Here's how the part is built. I have some questions about the finished solid (model axes, mm). A direction names the side the tool comes from. Round coordinates to 2 decimals unless told otherwise and drop trailing zeros. Loops run counter-clockwise (first coordinate to the right, second up) from the corner with the lowest first, then second, coordinate; pieces in that order, holes last. Notation, with made-up numbers: (35.25, 53) -> (77.25, 53) arc R22 ccw to (77.25, 68) -> close; hole circle Ø5 at (70, 4.5). An arc over 180 degrees is marked (long way). Use CSV: the item, a comma, the result in double quotes. Start each with the question number.
from build123d import *

# Parameters (mm, degrees)
F0_W     = 10.2
F0_H     = 10.2
F0_W_2   = 32
F0_H_2   = 26
F0_W_3   = 6
F0_H_3   = 6
F0_W_4   = 8
F0_H_4   = 7
F0_H_5   = 1
F1_DEPTH = 2
F2_DEPTH = 8.5
F3_DEPTH = 10.2
F4_DEPTH = 25
F6_DEPTH = 5.5


with BuildPart() as f1:
    # F0 (on Right) → F1 (new body)
    with BuildSketch(Plane.YZ):
        Polygon((0, 55), (0, 26), (32, 26), (32, 55), (30, 55), (30, 48), (22, 48), (22, 55), align=None)
        with Locations((21.9, 39.9)):
            Rectangle(F0_W, F0_H, mode=Mode.SUBTRACT)
        with Locations((16, 13)):
            Rectangle(F0_W_2, F0_H_2)
        with Locations((6.6, 12)):
            Rectangle(F0_W_3, F0_H_3, mode=Mode.SUBTRACT)
        with Locations((25.4, 12)):
            Rectangle(F0_W_3, F0_H_3, mode=Mode.SUBTRACT)
        Polygon((0, 60), (0, 55), (22, 55), (22, 56), (30, 56), (30, 55), (32, 55), (32, 60), align=None)
        with Locations((21.9, 39.9)):
            Rectangle(F0_W, F0_H)
        with Locations((26, 51.5)):
            Rectangle(F0_W_4, F0_H_4)
        with Locations((25.4, 12)):
            Rectangle(F0_W_3, F0_H_3)
        with Locations((6.6, 12)):
            Rectangle(F0_W_3, F0_H_3)
        with Locations((26, 55.5)):
            Rectangle(F0_W_4, F0_H_5)
    extrude(amount=F1_DEPTH)

    # F0 (on Right) → F2 (join)
    with BuildSketch(Plane.YZ):
        Polygon((0, 55), (0, 26), (32, 26), (32, 55), (30, 55), (30, 48), (22, 48), (22, 55), align=None)
        with Locations((21.9, 39.9)):
            Rectangle(F0_W, F0_H, mode=Mode.SUBTRACT)
        with Locations((26, 51.5)):
            Rectangle(F0_W_4, F0_H_4)
        with Locations((21.9, 39.9)):
            Rectangle(F0_W, F0_H)
    extrude(amount=-F2_DEPTH)

    # F0 (on Right) → F4 (join)
    with BuildSketch(Plane.YZ):
        with Locations((26, 51.5)):
            Rectangle(F0_W_4, F0_H_4)
        with Locations((26, 55.5)):
            Rectangle(F0_W_4, F0_H_5)
    extrude(amount=F4_DEPTH)


with BuildPart() as f3:
    # F0 (on Right) → F3 (new body)
    with BuildSketch(Plane.YZ):
        with Locations((21.9, 39.9)):
            Rectangle(F0_W, F0_H)
    extrude(amount=F3_DEPTH)

    # F5: union F1
    add(f1.part)

    # F0 (on Right) → F6 (join)
    with BuildSketch(Plane.YZ):
        with Locations((6.6, 12)):
            Rectangle(F0_W_3, F0_H_3)
        with Locations((25.4, 12)):
            Rectangle(F0_W_3, F0_H_3)
    extrude(amount=-F6_DEPTH)


solid = f3.part
Q1. Will these pins go through, and if not, where does the flat tip stop? pin 1 Ø1.6 at (x, y) = (-3.5, 26.5) entering from +Z; pin 2 Ø2.5 at (y, z) = (22, 58.5) entering from -X; pin 3 Ø3 at (y, z) = (13.5, 53) entering from +X; pin 4 Ø1.5 at (x, z) = (11, 40.5) entering from +Y.
Q2. For faces 4 (the flat face through (-3, 25, 9)), 5 (the flat face through (6, 16.8, 40)), 6 (the flat face through (-3, 3.6, 12)), 7 (the flat face through (-4, 16, 26)), 8 (the flat face through (10.2, 22, 40)), which set-ups out of +Z, -Z, +X, -X, +Y, -Y let a thin tool reach every point of the face, with its end or its side?
Q3. I want a section at C-C, the plane y = 18.5. List the corners of the cut face in (x, z) for me, then the cut area to 3 significant figures.
Q4. I want a section at B-B, the plane z = 50. List the corners of the cut face in (x, y) for me, then the cut area to 3 significant figures.
Q5. I need wall thicknesses on line 1 along Z through (x, y) = (-3, 28); line 2 along X through (y, z) = (6.5, 11.5); line 3 along X through (y, z) = (15, 25). Which ranges of each line are inside material? Lowest first, please.
Q6. I want a section at D-D, the plane z = 13. List the corners of the cut face in (x, y) for me.
Q7. I want a section at A-A, the plane x = 3. List the corners of the cut face in (y, z) for me, then the cut area to 3 significant figures.
Q8. If we mould it in two halves opening along Z, with no side actions, what happens to faces 1 (the flat face through (-3, 7, 15)), 2 (the flat face through (-5.5, 7, 12)), 3 (the flat face through (6, 22, 34.8))? For each: pulls with the +Z half, pulls with the -Z half, needs draft (parallel to the pull), parting line crosses it, or undercut.
Values found:
1,pin 1,"z = 55"
1,pin 2,"x = 0"
1,pin 3,"x = 2"
1,pin 4,"through"
2,face 4,"-Z, -X, +Y, -Y"
2,face 5,"+Z, -Z, +X, -Y"
2,face 6,"-Z, -X, -Y"
2,face 7,"-X, +Y, -Y"
2,face 8,"-Z, +X, +Y, -Y"
3,outline,"(-8.5, 26) -> (0, 26) -> (0, 0) -> (2, 0) -> (2, 34.8) -> (10.2, 34.8) -> (10.2, 45) -> (2, 45) -> (2, 60) -> (0, 60) -> (0, 55) -> (-8.5, 55) -> close"
3,area,"450 mm2"
4,outline,"(-8.5, 0) -> (2, 0) -> (2, 22) -> (25, 22) -> (25, 30) -> (2, 30) -> (2, 32) -> (-8.5, 32) -> close"
4,area,"520 mm2"
5,line 1,"9 to 15, 26 to 55"
5,line 2,"-5.5 to 2"
5,line 3,"0 to 2"
6,outline,"(-5.5, 3.6) -> (0, 3.6) -> (0, 0) -> (2, 0) -> (2, 32) -> (0, 32) -> (0, 28.4) -> (-5.5, 28.4) -> (-5.5, 22.4) -> (0, 22.4) -> (0, 9.6) -> (-5.5, 9.6) -> close"
7,outline,"(16.8, 34.8) -> (27, 34.8) -> (27, 45) -> (16.8, 45) -> close; (22, 48) -> (30, 48) -> (30, 56) -> (22, 56) -> close"
7,area,"168 mm2"
8,face 1,"undercut"
8,face 2,"needs draft"
8,face 3,"pulls with the -Z half"
